Could you check a few things on this model? Use its own coordinates, in mm. A direction names the side the tool comes from. Round coordinates to 2 decimals unless told otherwise and drop trailing zeros. Write each loop counter-clockwise with the first axis right and the second up, starting at its lowest first coordinate (ties: lowest second). Pieces come first, ordered by that corner, then holes. Notation, with made-up numbers: (-6, 38.5) - (12, 38.5) arc R13 cw to (12, 50.5) - close; hole circle Ø9 at (32.5, -37). An arc over 180 degrees is marked (long way). Put each result on its own line as item: value.
from build123d import *

# Parameters (mm, degrees)
SKETCH1_W                = 25
SKETCH1_H                = 25
BOSS_EXTRUDE1_DEPTH      = 3
M3_CLEARANCE_HOLE1_D     = 3.2
M3_CLEARANCE_HOLE1_DEPTH = 5
M3_CLEARANCE_HOLE1_TIP   = 0.96137699
SKETCH4_W                = 7
SKETCH4_H                = 4
CUT_EXTRUDE1_DEPTH       = 3
FILLET2_R                = 10


with BuildPart() as part:
    # Sketch1 → Boss-Extrude1 (new body)
    with BuildSketch(Plane(origin=(0, 0, 0), x_dir=(1, 0, 0), z_dir=(0, 1, 0))):
        Rectangle(SKETCH1_W, SKETCH1_H)
    extrude(amount=BOSS_EXTRUDE1_DEPTH)

    # M3 Clearance Hole1
    with Locations(Plane(origin=(-7.5, 3, 9.75), x_dir=(0, 0, 1), z_dir=(0, 1, 0))):
        with Locations((0, 0), (0, 15)):
            Hole(M3_CLEARANCE_HOLE1_D / 2, depth=M3_CLEARANCE_HOLE1_DEPTH)
            with Locations((0, 0, -(M3_CLEARANCE_HOLE1_DEPTH + M3_CLEARANCE_HOLE1_TIP / 2))):  # 118° drill point
                Cone(0, M3_CLEARANCE_HOLE1_D / 2, M3_CLEARANCE_HOLE1_TIP, mode=Mode.SUBTRACT)

    # Sketch4 → Cut-Extrude1 (cut)
    with BuildSketch(Plane(origin=(0, 3, 0), x_dir=(1, 0, 0), z_dir=(0, 1, 0))):
        with Locations((0, 1.5)):
            Rectangle(SKETCH4_W, SKETCH4_H)
    extrude(amount=-CUT_EXTRUDE1_DEPTH, mode=Mode.SUBTRACT)

    # Fillet2
    # the kernel refuses this fillet: 10 mm, written as the material it takes off along each edge
    with BuildSketch(Plane(origin=(3.5, 3, 0.5), x_dir=(1, 0, 0), z_dir=(0, 0, -1)), Plane(origin=(-3.5, 3, -3.5), x_dir=(-1, 0, 0), z_dir=(0, 0, 1))) as fillet2_piece_1:
        with BuildLine():
            CenterArc((7.141428429, 10), FILLET2_R, 224.427004001, 45.572995999)
            Line((0, 3), (0, 0))
            Line((0, 0), (7.141428429, 0))
        make_face()
    extrude(amount=4, mode=Mode.SUBTRACT)
    with BuildSketch(Plane(origin=(3.5, 3, -3.5), x_dir=(0, 0, -1), z_dir=(-1, 0, 0)), Plane(origin=(-3.5, 3, 0.5), x_dir=(0, 0, 1), z_dir=(1, 0, 0))) as fillet2_piece_2:
        with BuildLine():
            CenterArc((7.141428429, 10), FILLET2_R, 224.427004001, 45.572995999)
            Line((0, 3), (0, 0))
            Line((0, 0), (7.141428429, 0))
        make_face()
    extrude(amount=7, mode=Mode.SUBTRACT)
    with BuildSketch(Plane(origin=(-3.5, 3, 0.5), x_dir=(0, 0, 1), z_dir=(1, 0, 0))) as fillet2_piece_3a_section:
        with BuildLine():
            CenterArc((7.141428429, 10), FILLET2_R, 224.427004001, 45.572995999)
            Line((0, 3), (0, 0))
            Line((0, 0), (7.141428429, 0))
        make_face()
    fillet2_piece_3a = extrude(amount=24.853571071, mode=Mode.PRIVATE)
    fillet2_piece_3a = split(fillet2_piece_3a, bisect_by=Plane(origin=(12.5, 3, 0.5), z_dir=(-1, 0, 0)), keep=Keep.TOP, mode=Mode.PRIVATE)
    fillet2_piece_3a = split(fillet2_piece_3a, bisect_by=Plane(origin=(3.5, 3, 0.5), z_dir=(1, 0, 0)), keep=Keep.TOP, mode=Mode.PRIVATE)
    with BuildSketch(Plane(origin=(3.5, 3, 18.353571071), x_dir=(1, 0, 0), z_dir=(0, 0, -1))) as fillet2_piece_3b_section:
        with BuildLine():
            CenterArc((7.141428429, 10), FILLET2_R, 224.427004001, 45.572995999)
            Line((0, 3), (0, 0))
            Line((0, 0), (7.141428429, 0))
        make_face()
    fillet2_piece_3b = extrude(amount=21.853571071, mode=Mode.PRIVATE)
    fillet2_piece_3b = split(fillet2_piece_3b, bisect_by=Plane(origin=(3.5, 3, 12.5), z_dir=(0, 0, -1)), keep=Keep.TOP, mode=Mode.PRIVATE)
    fillet2_piece_3b = fillet2_piece_3b - Plane(origin=(7.5, 3, 9.75), x_dir=(0, 0, -1), z_dir=(0, -1, 0)) * Cylinder(1.6, 73, mode=Mode.PRIVATE)
    fillet2_piece_3b = split(fillet2_piece_3b, bisect_by=Plane(origin=(3.5, 3, 0.5), z_dir=(0, 0, 1)), keep=Keep.TOP, mode=Mode.PRIVATE)
    fillet2_piece_3 = fillet2_piece_3a & fillet2_piece_3b
    add(fillet2_piece_3, mode=Mode.SUBTRACT)
    with BuildSketch(Plane(origin=(3.5, 3, 0.5), x_dir=(1, 0, 0), z_dir=(0, 0, -1))) as fillet2_piece_4a_section:
        with BuildLine():
            CenterArc((7.141428429, 10), FILLET2_R, 224.427004001, 45.572995999)
            Line((0, 3), (0, 0))
            Line((0, 0), (7.141428429, 0))
        make_face()
    fillet2_piece_4a = extrude(amount=21.853571071, mode=Mode.PRIVATE)
    fillet2_piece_4a = split(fillet2_piece_4a, bisect_by=Plane(origin=(3.5, 3, -12.5), z_dir=(0, 0, 1)), keep=Keep.TOP, mode=Mode.PRIVATE)
    fillet2_piece_4a = split(fillet2_piece_4a, bisect_by=Plane(origin=(3.5, 3, -3.5), z_dir=(0, 0, -1)), keep=Keep.TOP, mode=Mode.PRIVATE)
    with BuildSketch(Plane(origin=(21.353571071, 3, -3.5), x_dir=(0, 0, -1), z_dir=(-1, 0, 0))) as fillet2_piece_4b_section:
        with BuildLine():
            CenterArc((7.141428429, 10), FILLET2_R, 224.427004001, 45.572995999)
            Line((0, 3), (0, 0))
            Line((0, 0), (7.141428429, 0))
        make_face()
    fillet2_piece_4b = extrude(amount=24.853571071, mode=Mode.PRIVATE)
    fillet2_piece_4b = split(fillet2_piece_4b, bisect_by=Plane(origin=(12.5, 3, -3.5), z_dir=(-1, 0, 0)), keep=Keep.TOP, mode=Mode.PRIVATE)
    fillet2_piece_4b = split(fillet2_piece_4b, bisect_by=Plane(origin=(3.5, 3, -3.5), z_dir=(1, 0, 0)), keep=Keep.TOP, mode=Mode.PRIVATE)
    fillet2_piece_4 = fillet2_piece_4a & fillet2_piece_4b
    add(fillet2_piece_4, mode=Mode.SUBTRACT)
    with BuildSketch(Plane(origin=(3.5, 3, -3.5), x_dir=(0, 0, -1), z_dir=(-1, 0, 0))) as fillet2_piece_5a_section:
        with BuildLine():
            CenterArc((7.141428429, 10), FILLET2_R, 224.427004001, 45.572995999)
            Line((0, 3), (0, 0))
            Line((0, 0), (7.141428429, 0))
        make_face()
    fillet2_piece_5a = extrude(amount=24.853571071, mode=Mode.PRIVATE)
    fillet2_piece_5a = split(fillet2_piece_5a, bisect_by=Plane(origin=(-12.5, 3, -3.5), z_dir=(1, 0, 0)), keep=Keep.TOP, mode=Mode.PRIVATE)
    fillet2_piece_5a = split(fillet2_piece_5a, bisect_by=Plane(origin=(-3.5, 3, -3.5), z_dir=(-1, 0, 0)), keep=Keep.TOP, mode=Mode.PRIVATE)
    with BuildSketch(Plane(origin=(-3.5, 3, -21.353571071), x_dir=(-1, 0, 0), z_dir=(0, 0, 1))) as fillet2_piece_5b_section:
        with BuildLine():
            CenterArc((7.141428429, 10), FILLET2_R, 224.427004001, 45.572995999)
            Line((0, 3), (0, 0))
            Line((0, 0), (7.141428429, 0))
        make_face()
    fillet2_piece_5b = extrude(amount=21.853571071, mode=Mode.PRIVATE)
    fillet2_piece_5b = split(fillet2_piece_5b, bisect_by=Plane(origin=(-3.5, 3, -12.5), z_dir=(0, 0, 1)), keep=Keep.TOP, mode=Mode.PRIVATE)
    fillet2_piece_5b = split(fillet2_piece_5b, bisect_by=Plane(origin=(-3.5, 3, -3.5), z_dir=(0, 0, -1)), keep=Keep.TOP, mode=Mode.PRIVATE)
    fillet2_piece_5 = fillet2_piece_5a & fillet2_piece_5b
    add(fillet2_piece_5, mode=Mode.SUBTRACT)
    with BuildSketch(Plane(origin=(-21.353571071, 3, 0.5), x_dir=(0, 0, 1), z_dir=(1, 0, 0))) as fillet2_piece_6a_section:
        with BuildLine():
            CenterArc((7.141428429, 10), FILLET2_R, 224.427004001, 45.572995999)
            Line((0, 3), (0, 0))
            Line((0, 0), (7.141428429, 0))
        make_face()
    fillet2_piece_6a = extrude(amount=24.853571071, mode=Mode.PRIVATE)
    fillet2_piece_6a = split(fillet2_piece_6a, bisect_by=Plane(origin=(-12.5, 3, 0.5), z_dir=(1, 0, 0)), keep=Keep.TOP, mode=Mode.PRIVATE)
    fillet2_piece_6a = split(fillet2_piece_6a, bisect_by=Plane(origin=(-3.5, 3, 0.5), z_dir=(-1, 0, 0)), keep=Keep.TOP, mode=Mode.PRIVATE)
    with BuildSketch(Plane(origin=(-3.5, 3, -3.5), x_dir=(-1, 0, 0), z_dir=(0, 0, 1))) as fillet2_piece_6b_section:
        with BuildLine():
            CenterArc((7.141428429, 10), FILLET2_R, 224.427004001, 45.572995999)
            Line((0, 3), (0, 0))
            Line((0, 0), (7.141428429, 0))
        make_face()
    fillet2_piece_6b = extrude(amount=21.853571071, mode=Mode.PRIVATE)
    fillet2_piece_6b = split(fillet2_piece_6b, bisect_by=Plane(origin=(-3.5, 3, 12.5), z_dir=(0, 0, -1)), keep=Keep.TOP, mode=Mode.PRIVATE)
    fillet2_piece_6b = fillet2_piece_6b - Plane(origin=(-7.5, 3, 9.75), x_dir=(0, 0, -1), z_dir=(0, -1, 0)) * Cylinder(1.6, 73, mode=Mode.PRIVATE)
    fillet2_piece_6b = split(fillet2_piece_6b, bisect_by=Plane(origin=(-3.5, 3, 0.5), z_dir=(0, 0, 1)), keep=Keep.TOP, mode=Mode.PRIVATE)
    fillet2_piece_6 = fillet2_piece_6a & fillet2_piece_6b
    add(fillet2_piece_6, mode=Mode.SUBTRACT)


solid = part.part
(1) Imagine slicing it at D-D, the plane z = -7. List the corners of the cut face in (x, y) for me.
Values found:
outline: (-12.5, 0) - (12.5, 0) - (12.5, 3) - (10.64, 3) arc R10 ccw to (7, 2.31) - (-7, 2.31) arc R10 ccw to (-10.64, 3) - (-12.5, 3) - close
(2) For faces 4 (the face through (7.544, 2.508, -1.372)), 5 (the face through (12.5, 1, 0)), which set-ups out of +Z, -Z, +X, -X, +Y, -Y let a thin tool reach every point of the face, with its end or its side?
Values found:
face 4: +Y
face 5: +Z, -Z, +X, +Y, -Y
(3) Imagine slicing it at B-B, the plane x = -2. List the corners of the cut face in (y, z) for me, then the cut area to 3 significant figures.
Values found:
outline: (0, -12.5) - (3, -12.5) - (3, -10.64) arc R10 ccw to (0, -3.5) - close; (0, 0.5) arc R10 ccw to (3, 7.64) - (3, 12.5) - (0, 12.5) - close
area: 49.7 mm^2
(4) If we mould it in two halves opening along Z, with no side actions, what happens to faces 1 (the face through (0, 1, 12.5)), 2 (the face through (-7.544, 2.508, -1.628)), 3 (the face through (-12.5, 1, 0))? For each: pulls with the +Z half, pulls with the -Z half, needs draft (parallel to the pull), parting line crosses it, or undercut.
Values found:
face 1: pulls with the +Z half
face 2: undercut
face 3: needs draft
(5) Imagine slicing it at C-C, the plane y = 1.8. List the corners of the cut face in (x, z) for me.
Values found:
outline: (-12.5, -12.5) - (12.5, -12.5) - (12.5, 12.5) - (-12.5, 12.5) - close; hole circle Ø3.2 at (-7.5, 9.75); hole (-5.89, -5.89) - (5.89, -5.89) - (5.89, 2.89) - (-5.89, 2.89) - close; hole circle Ø3.2 at (7.5, 9.75)
(6) I'm going to push a flat-ended pin straight in: pin 1 (1.9 mm diameter, centred on x = -7.5, z = 9.75, fed in from +Y). Where does the tip first touch, or does it pass through?
Values found:
pin 1: passes through
(7) Please list where these lines run through material, in increasing order: probe 1 along X at (y, z) = (2.3, 9.75); probe 2 along X at (y, z) = (2.85, 10.5); probe 3 along Z at (x, y) = (0.75, 2.1). Write a range as from..to.
Values found:
probe 1: x = -12.5..-9.1, -5.9..5.9, 9.1..12.5
probe 2: x = -12.5..-8.91, -6.09..6.09, 8.91..12.5
probe 3: z = -12.5..-6.5, 3.5..12.5
(8) Imagine slicing it at A-A, the plane z = 9.75. List the corners of the cut face in (x, y) for me, then the cut area to 3 significant figures.
Values found:
outline: (-12.5, 0) - (-9.1, 0) - (-9.1, 3) - (-12.5, 3) - close; (-5.9, 0) - (5.9, 0) - (5.9, 3) - (-5.9, 3) - close; (9.1, 0) - (12.5, 0) - (12.5, 3) - (9.1, 3) - close
area: 55.8 mm^2
